Geometry check sheet. Reference: the model listing, model coordinates, mm. Coordinates: 2 decimals unless noted, no trailing zeros. Loops run counter-clockwise (first coordinate to the right, second up) from the corner with the lowest first, then second, coordinate; pieces in that order, holes last.
Autodesk Inventor part; units mm, degrees
ref_plane "YZ Plane" through (0, 0, 0) normal (1, 0, 0) x (0, 1, 0)
ref_plane "XZ Plane" through (0, 0, 0) normal (0, 1, 0) x (-1, 0, 0)
ref_plane "XY Plane" through (0, 0, 0) normal (0, 0, 1) x (1, 0, 0)
sketch "Skizze1" plane through (0, 0, 0) normal (0, 1, 0) x (-1, 0, 0)
  line L0 (0, 3) -> (0, 5)
  line L1 (0, 5) -> (-125, 5)
  line L2 (-125, 5) -> (-125, 0)
  line L3 (-125, 0) -> (-10, 0)
  line L4 (-10, 0) -> (0, 3)
  point P0 (0, 0)
  dimension "d0" = 10
  dimension "d1" = 2
  dimension "d2" = 125
  dimension "d3" = 5
extrude "Extrusion1" add sketch "Skizze1" along normal blind 14
sketch "Skizze2" plane through (0, 0, 5) normal (0, 0, 1) x (1, 0, 0)
  line L0 (0, 0) -> (0, 14)
  point P0 (24, 7)
  point P1 (0, 7)
  dimension "d13" = 24
hole "Bohrung1" at (24, 7, 5) direction (0, 0, -1) diameter 3.242 depth 5
sketch "Skizze3" plane through (0, 0, 5) normal (0, 0, 1) x (1, 0, 0)
  circle A0 centre (24, 7) radius 1.621
  line L0 (0, 0) -> (0, 14)
  point P0 (67, 7)
  point P1 (0, 7)
  dimension "d21" = 43
hole "Bohrung2" at (67, 7, 5) direction (0, 0, -1) diameter 4.917 end through all
sketch "Skizze4" plane through (0, 0, 5) normal (0, 0, 1) x (1, 0, 0)
  line L0 (0, 0) -> (0, 14)
  circle A0 centre (67, 7) radius 2.4585
  line L1 (125, 0) -> (125, 14)
  point P0 (119, 7)
  point P1 (0, 7)
  point P2 (125, 7)
  dimension "d29" = 52
  dimension "d30" = 6
hole "Bohrung3" at (119, 7, 5) direction (0, 0, -1) diameter 4 end through all
chamfer "Fasen1" distance 0.2 angle 45 9 edges at (62.5, 0, 5) (62.5, 14, 5) (125, 7, 5) (125, 0, 2.5) (67.5, 0, 0) (125, 7, 0) (125, 14, 2.5) (67.5, 14, 0) (0, 7, 5)
properties part number "112"
(1) Sectioned sample at B-B on y = 7. Record the cut outline in (x, z), and give its area (3 significant figures).
Findings:
outline: (0, 3) - (10, 0) - (22.38, 0) - (22.38, 5) - (0.2, 5) - (0, 4.8) - close; (25.62, 0) - (64.54, 0) - (64.54, 5) - (25.62, 5) - close; (69.46, 0) - (117, 0) - (117, 5) - (69.46, 5) - close; (121, 0) - (124.8, 0) - (125, 0.2) - (125, 4.8) - (124.8, 5) - (121, 5) - close
area: 549 mm2
(2) Sectioned sample at D-D on y = 2.5. Record the cut outline in (x, z).
Findings:
outline: (0, 3) - (10, 0) - (124.8, 0) - (125, 0.2) - (125, 4.8) - (124.8, 5) - (0.2, 5) - (0, 4.8) - close
(3) Scan lines: L1, parallel to X at y = 7, z = 3.6; L2, parallel to Y at x = 24, z = 1.5; L3, parallel to Y at x = 67, z = 1.25. Record each from-to range of solid material in increasing order.
Findings:
L1: x = 0 to 22.38, 25.62 to 64.54, 69.46 to 117, 121 to 125
L2: y = 0 to 5.38, 8.62 to 14
L3: y = 0 to 4.54, 9.46 to 14
(4) Sectioned sample at A-A on x = 67. Record the cut outline in (y, z).
Findings:
outline: (0, 0.2) - (0.2, 0) - (4.54, 0) - (4.54, 5) - (0.2, 5) - (0, 4.8) - close; (9.46, 0) - (13.8, 0) - (14, 0.2) - (14, 4.8) - (13.8, 5) - (9.46, 5) - close
(5) Gauge pin test, flat end, axial feed: pin 1 Ø1.9 at (x, y) = (24, 7) entering from -Z. Record the tip position at first contact, or that the pin passes through.
Findings:
pin 1: passes through
(6) Sectioned sample at C-C on x = 119. Record the cut outline in (y, z), and give its area (3 significant figures).
Findings:
outline: (0, 0.2) - (0.2, 0) - (5, 0) - (5, 5) - (0.2, 5) - (0, 4.8) - close; (9, 0) - (13.8, 0) - (14, 0.2) - (14, 4.8) - (13.8, 5) - (9, 5) - close
area: 49.9 mm2
(7) Draft check along Y on faces 1 (the flat face through (68, 4, 0)), 2 (the cylindrical face through (117.314, 5.925, 2.465)), 3 (the flat face through (63, 14, 3)). Enter one of: +Y half, -Y half, draft (parallel to the pull), parting line (faces both ways), or undercut.
Findings:
face 1: draft
face 2: undercut
face 3: +Y half
